from build123d import *

# Parameters (mm, degrees)
SKETCH1_R           = 45
BOSS_EXTRUDE1_DEPTH = 55
SKETCH7_R           = 4
CUT_EXTRUDE1_DEPTH  = 15


with BuildPart() as part:
    # Sketch1 → Boss-Extrude1 (new body)
    with BuildSketch(Plane(origin=(0, 0, 0), x_dir=(1, 0, 0), z_dir=(0, 1, 0))):
        with Locations(Location((0, 0, 0), (0, 0, 270))):
            Circle(SKETCH1_R)
    extrude(amount=BOSS_EXTRUDE1_DEPTH)

    # Sketch6 → Cut-Revolve2 (revolve, cut)
    with BuildSketch(Plane(origin=(0, 0, 0), x_dir=(0, 0, -1), z_dir=(1, 0, 0))):
        Polygon((0, 55), (0, 35), (-25, 35), (-35, 55), align=None)
        Polygon((0, 0), (0, 20), (-25, 20), (-35, 0), align=None)
    revolve(axis=Axis((0, 57.084701854, 0), (0, -1, 0)), mode=Mode.SUBTRACT)

    # Sketch7 → Cut-Extrude1 (cut)
    with BuildSketch(Plane(origin=(0, 35, 0), x_dir=(1, 0, 0), z_dir=(0, 1, 0))):
        with Locations(Location((0, 0, 0), (0, 0, 270))):
            Circle(SKETCH7_R)
    extrude(amount=-CUT_EXTRUDE1_DEPTH, mode=Mode.SUBTRACT)


solid = part.part
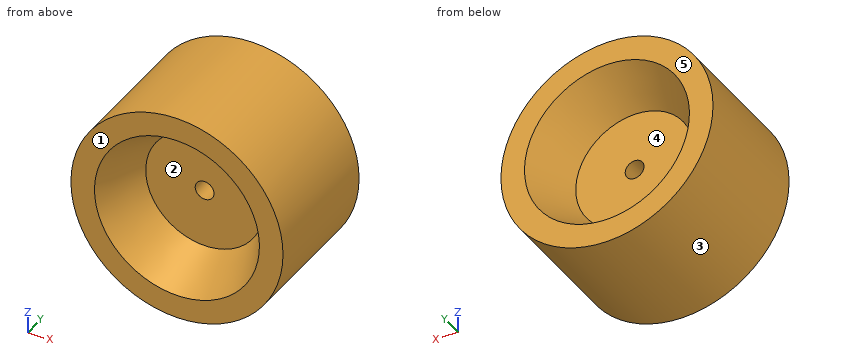
Work out the finished part from the listing and answer in its coordinate system (mm). Face numbers are marked on the shaded views. A direction names the side the tool comes from. Coordinates: 2 decimals unless noted, no trailing zeros. Write each loop counter-clockwise with the first axis right and the second up, starting at its lowest first coordinate (ties: lowest second). Pieces come first, ordered by that corner, then holes. Notation, with made-up numbers: M -1.75,84 L 13.25,84 A24 ccw 13.25,98 Z; hole C -13,-31.5 d11. An arc over 180 degrees is marked long. Answer as CSV lines item,"result". Start each with the question number.
Item 1: Section A-A on z = 0 is taken. Write down the section's boundary in (x, y).
Item 2: Section C-C on y = 26 is taken. Write down the section's boundary in (x, z).
Item 3: Section D-D on z = 38 is taken. Write down the section's boundary in (x, y).
Item 4: Section B-B on x = 0 is taken. Write down the section's boundary in (y, z).
Item 5: Consider L1, parallel to X at y = 30, z = 0; L2, parallel to Y at x = 0.5, z = -22.5; L3, parallel to Z at x = -20, y = 4. Determine where each line is inside the solid, lowest interval first.
Item 6: A tool of negligible diameter and unlimited length cuts with its end or side. For the marked faces 4 and 5, from which of +Z, -Z, +X, -X, +Y, -Y can it reach the whole face along a straight path? Write none if from no direction.
Item 7: Determine the mould class of the marked faces 1, 2 and 3 for opening direction X: released by +X, released by -X, zero draft, split by the parting line, or undercut.
Item 8: Flat-ended cylindrical pins translate along their axes: P1, Ø5, axis at x = -26.5, y = 31, coming from the -Z side; P2, Ø10.5, axis at x = 0, z = 0, coming from the -Y side; P3, Ø12, axis at x = 2.5, z = -11, coming from the +Y side; P4, Ø5, axis at x = 33.5, z = -6.5, coming from the -Y side. Find the tip coordinate at first contact, or state that the pin passes through.
Checks:
1,outline,"M -45,0 L -35,0 L -25,20 L -4,20 L -4,35 L -25,35 L -35,55 L -45,55 Z; M 4,20 L 25,20 L 35,0 L 45,0 L 45,55 L 35,55 L 25,35 L 4,35 Z"
2,outline,"C 0,0 d90; hole C 0,0 d8"
3,outline,"M -24.1,0 L 24.1,0 L 24.1,55 L -24.1,55 Z"
4,outline,"M 0,-45 L 55,-45 L 55,-35 L 35,-25 L 35,-4 L 20,-4 L 20,-25 L 0,-35 Z; M 0,35 L 20,25 L 20,4 L 35,4 L 35,25 L 55,35 L 55,45 L 0,45 Z"
5,L1,"x = -45 to -4, 4 to 45"
5,L2,"y = 20 to 35"
5,L3,"z = -40.31 to -26.25, 26.25 to 40.31"
6,face 4,"+Y"
6,face 5,"+Z, -Z, +X, -X, +Y"
7,face 1,"zero draft"
7,face 2,"undercut"
7,face 3,"split by the parting line"
8,P1,"stops at z = -38.07"
8,P2,"stops at y = 20"
8,P3,"stops at y = 35"
8,P4,"stops at y = 0"
